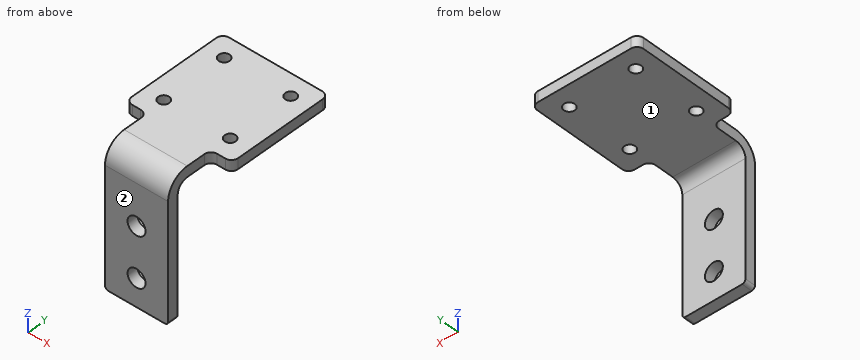
Autodesk Inventor part; units mm, degrees
ref_plane "YZ Plane" through (0, 0, 0) normal (1, 0, 0) x (0, 1, 0)
ref_plane "XZ Plane" through (0, 0, 0) normal (0, 1, 0) x (-1, 0, 0)
ref_plane "XY Plane" through (0, 0, 0) normal (0, 0, 1) x (1, 0, 0)
sketch "Sketch1" plane through (0, 0, 0) normal (0, 0, 1) x (1, 0, 0)
  line L0 (16, -16) -> (-16, -16)
  line L1 (-16, -16) -> (-16, 16)
  line L2 (-16, 16) -> (16, 16)
  line L3 (16, 16) -> (16, -16)
  line L4 (16, -16) -> (-16, 16) construction
  line L5 (-16, -16) -> (16, 16) construction
  line L6 (10, -10) -> (-10, -10) construction
  line L7 (-10, -10) -> (-10, 10) construction
  line L8 (-10, 10) -> (10, 10) construction
  line L9 (10, 10) -> (10, -10) construction
  line L10 (10, -10) -> (-10, 10) construction
  line L11 (-10, -10) -> (10, 10) construction
  line L12 (-9.5, -16) -> (9.5, -16)
  line L13 (9.5, -16) -> (9.5, -30)
  line L14 (9.5, -30) -> (-9.5, -30)
  line L15 (-9.5, -30) -> (-9.5, -16)
  point P0 (0, 0)
  point P1 (0, -16)
  dimension "d0" = 32
  dimension "d1" = 32
  dimension "d2" = 20
  dimension "d3" = 20
  dimension "d4" = 19
  dimension "d5" = 30
extrude "Plate1" add sketch "Sketch1" along normal blind 3.175
sketch "Sketch2" plane through (-9.5, -26.825, 3.175) normal (0, -1, 0) x (1, 0, 0)
  line L0 (19, 0) -> (0, 0)
  line L1 (0, 0) -> (0, -50)
  line L2 (0, -50) -> (19, -50)
  line L3 (19, -50) -> (19, 0)
edge flange "Flange1" height 50 angle 90 thickness 3.175 bend radius 3.175 thickness toward (0, -1, 0) relief tear relief width 3.175 relief depth 1.5875 edges at (0, -30, 0) wall of the first edge with corners at (9.5, -26.825, 3.175) (-9.5, -26.825, 3.175) (-9.5, -26.825, -46.825) (9.5, -26.825, -46.825)
bend "Bend1"
corner "Corner1"
fillet "Fillet1" radius 2 6 edges at (-16, -16, 1.5875) (-16, 16, 1.5875) (16, 16, 1.5875) (16, -16, 1.5875) (9.5, -16, 1.5875) (-9.5, -16, 1.5875)
hole "Hole1" at (10, -10, 0) at (10, 10, 0) at (-10, 10, 0) at (-10, -10, 0) direction (0, 0, 1) diameter 3.3 end through all
sketch "Sketch3" plane through (-9.5, -30, -46.825) normal (0, -1, 0) x (1, 0, 0)
  line L0 (1.15, 46.825) -> (-2.15, 46.825) construction
  line L1 (1.15, 46.825) -> (-2.15, 46.825) construction
  line L2 (21.15, 46.825) -> (17.85, 46.825) construction
  line L3 (21.15, 46.825) -> (17.85, 46.825) construction
  line L4 (23.5, 46.825) -> (25.5, 46.825) construction
  line L5 (21, 46.825) -> (23.5, 46.825) construction
  line L6 (19, 46.825) -> (21, 46.825) construction
  line L7 (19, 46.825) -> (0, 46.825) construction
  line L8 (-2, 46.825) -> (0, 46.825) construction
  line L9 (-4.5, 46.825) -> (-2, 46.825) construction
  line L10 (-6.5, 46.825) -> (-4.5, 46.825) construction
  line L11 (-4.5, 46.825) -> (-6.5, 46.825) construction
  line L12 (23.5, 46.825) -> (-4.5, 46.825) construction
  line L13 (25.5, 46.825) -> (23.5, 46.825) construction
  line L14 (0, 0) -> (0, 43.65) construction
  line L15 (19, 24.975) -> (0, 24.975) construction
  line L16 (0, 24.975) -> (0, 37.675) construction
  line L17 (0, 37.675) -> (19, 37.675) construction
  line L18 (19, 37.675) -> (19, 24.975) construction
  line L19 (19, 24.975) -> (0, 37.675) construction
  line L20 (0, 24.975) -> (19, 37.675) construction
  line L21 (19, 43.65) -> (19, 0) construction
  line L22 (0, 33.825) -> (19, 33.825) construction
  line L23 (19, 33.825) -> (19, 13.825) construction
  line L24 (19, 13.825) -> (0, 13.825) construction
  line L25 (0, 13.825) -> (0, 33.825) construction
  line L26 (19, 9.975) -> (0, 9.975) construction
  line L27 (0, 9.975) -> (0, 22.675) construction
  line L28 (0, 22.675) -> (19, 22.675) construction
  line L29 (19, 22.675) -> (19, 9.975) construction
  line L30 (19, 9.975) -> (0, 22.675) construction
  line L31 (0, 9.975) -> (19, 22.675) construction
  line L32 (0, 33.825) -> (19, 13.825) construction
  line L33 (0, 13.825) -> (19, 33.825) construction
  line L34 (19, 43.65) -> (0, 43.65)
  line L35 (0, 0) -> (0, 43.65)
  line L36 (19, 0) -> (0, 0)
  line L37 (19, 43.65) -> (19, 0)
  line L38 (0, 7.975) -> (19, 7.975)
  point P0 (9.5, 46.825)
  point P1 (9.5, 31.325)
  point P2 (9.5, 46.825)
  point P3 (9.5, 16.325)
  point P4 (9.5, 23.825)
  point P5 (9.5, 23.825)
  point P6 (19, 9.975)
  point P7 (0, 9.975)
  dimension "d25" = 12.7
  dimension "d27" = 20
  dimension "d28" = 13
  dimension "d29" = 7.5
  dimension "d30" = 7.5
  dimension "d33" = 2
extrude "Extrusion1" cut sketch "Sketch3" against normal through all contours L37 L36 L35 L38
fillet "Fillet2" radius 1 2 edges at (9.5, -28.4125, -38.85) (-9.5, -28.4125, -38.85)
hole "Hole2" at (0, -30, -15.5) at (0, -30, -30.5) direction (0, 1, 0) diameter 5.4 end through all
equation "\"d23\" = Thickness"
equation "\"d6\" = Thickness"
equation "\"d7\" = BendReliefWidth"
equation "\"d8\" = BendReliefDepth"
equation "\"d9\" = MinimumRemnant"
equation "\"d10\" = TransitionRadius"
equation "\"d13\" = BendRadius"
equation "\"d14\" = CornerReliefSize"
equation "\"d15\" = GapSize"
equation "\"d16\" = JacobiRadiusSize"
equation "\"BendReliefWidth\" = Thickness"
equation "\"BendReliefDepth\" = 0.5 * Thickness"
equation "\"CornerReliefSize\" = 4 * Thickness"
equation "\"MinimumRemnant\" = 2 * Thickness"
equation "\"TransitionRadius\" = BendRadius"
equation "\"JacobiRadiusSize\" = BendRadius"
equation "\"GapSize\" = Thickness"
properties part number "Printhead Belt Retainer Bracket" material "Aluminum 6061"
CAD build for the part. Positions are in the model's coordinates, mm. Face numbers are marked on the shaded views. A direction names the side the tool comes from. Round coordinates to 2 decimals unless told otherwise and drop trailing zeros. Order: outer loops, then holes, each group sorted by start corner. A loop starts at its lowest first (then second) coordinate and runs counter-clockwise, first axis right, second up. Notation, with made-up numbers: (-6, 84.5) - (41, 84.5) arc R15 ccw to (41, 93.5) - close; hole circle Ø9 at (7.25, -26). An arc over 180 degrees is marked (long way). Return JSON: item names as keys, results as strings.
(1) Cut at A-A (y = 10). Give the cut face in (x, z) (3 decimals).
Answer key:
{"outline": "(-16, 0) - (-11.65, 0) - (-11.65, 3.175) - (-16, 3.175) - close; (-8.35, 0) - (8.35, 0) - (8.35, 3.175) - (-8.35, 3.175) - close; (11.65, 0) - (16, 0) - (16, 3.175) - (11.65, 3.175) - close"}
(2) Wall check: probe 1 along X at (y, z) = (-10, 2.4); probe 2 along Y at (x, z) = (10, 2); probe 3 along X at (y, z) = (-28, -15.5). Give the ranges that are in metal, low to high. Write a range as from..to.
Answer key:
{"probe 1": "x = -16..-11.65, -8.35..8.35, 11.65..16", "probe 2": "y = -16.68..-11.65, -8.35..8.35, 11.65..16", "probe 3": "x = -9.5..-2.7, 2.7..9.5"}
(3) Tool access for the marked faces 1 and 2: list every direction of +Z, -Z, +X, -X, +Y, -Y with a clear straight run to the whole face (end or side of a thin tool).
Answer key:
{"face 1": "-Z, +X, -X, +Y", "face 2": "+Z, -Z, +X, -X, -Y"}
(4) Cut at D-D (x = -4). Give the cut face in (y, z) (3 decimals), then the cut area to 3 significant figures.
Answer key:
{"outline": "(-30, -38.85) - (-26.825, -38.85) - (-26.825, -3.175) arc R3.175 cw to (-23.65, 0) - (16, 0) - (16, 3.175) - (-23.65, 3.175) arc R6.35 ccw to (-30, -3.175) - close", "area": "263 mm^2"}
(5) Pin check, flat tips, straight feed: pin 1 Ø4 at (x, y) = (-10, 10) entering from +Z (3 decimals); pin 2 Ø6 at (x, y) = (12, 2) entering from -Z; pin 3 Ø4.5 at (x, z) = (0, -15.5) entering from -Y (1 decimal); pin 4 Ø6 at (x, z) = (11.5, -21.5) entering from +Y (3 decimals). Stop position of each tip, or through.
Answer key:
{"pin 1": "stops at z = 3.175", "pin 2": "stops at z = 0", "pin 3": "passes through", "pin 4": "stops at y = -26.825"}
(6) Cut at C-C (z = -30.5). Give the cut face in (x, y) (3 decimals).
Answer key:
{"outline": "(-9.5, -30) - (-2.7, -30) - (-2.7, -26.825) - (-9.5, -26.825) - close; (2.7, -30) - (9.5, -30) - (9.5, -26.825) - (2.7, -26.825) - close"}
(7) Cut at B-B (x = 0). Give the cut face in (y, z) (3 decimals).
Answer key:
{"outline": "(-30, -38.85) - (-26.825, -38.85) - (-26.825, -33.2) - (-30, -33.2) - close; (-30, -27.8) - (-26.825, -27.8) - (-26.825, -18.2) - (-30, -18.2) - close; (-30, -12.8) - (-26.825, -12.8) - (-26.825, -3.175) arc R3.175 cw to (-23.65, 0) - (16, 0) - (16, 3.175) - (-23.65, 3.175) arc R6.35 ccw to (-30, -3.175) - close"}
